Autodesk Inventor part; units mm, degrees
ref_plane "YZ Plane" through (0, 0, 0) normal (1, 0, 0) x (0, 1, 0)
ref_plane "XZ Plane" through (0, 0, 0) normal (0, 1, 0) x (-1, 0, 0)
ref_plane "XY Plane" through (0, 0, 0) normal (0, 0, 1) x (1, 0, 0)
sketch "Sketch1" plane through (0, 0, 0) normal (0, 1, 0) x (-1, 0, 0)
  line L0 (35, 45.5) -> (35, 15.5)
  line L1 (9, 15.5) -> (35, 15.5) construction
  line L2 (0, 15.5) -> (9, 15.5) construction
  line L3 (35, 15.5) -> (48, 15.5)
  line L4 (0, -45.5) -> (0, 45.5)
  line L5 (0, -45.5) -> (48, -45.5)
  line L6 (0, 45.5) -> (35, 45.5)
  line L7 (48, -45.5) -> (48, 15.5)
  line L8 (30.7, 40.55) -> (35, 40.55) construction
  line L9 (30.7, 40.55) -> (30.7, 22.45) construction
  circle A0 centre (30.7, 22.45) radius 1.25
  circle A1 centre (30.7, 40.55) radius 1.25
  line L10 (30.7, 22.45) -> (30.7, 15.5) construction
  line L11 (44, 15.5) -> (44, 9.5) construction
  line L12 (44, 9.5) -> (48, 9.5) construction
  circle A2 centre (44, 9.5) radius 1.25
  circle A3 centre (44, -28.5) radius 1.25
  circle A4 centre (18, -28.5) radius 1.25
  circle A5 centre (18, -38.5) radius 1.25
  arc A6 (0, -18.75) -> (0, -16.25) centre (0, -17.5) ccw
  arc A7 (0, 40.55) -> (0, 43.05) centre (0, 41.8) ccw
  arc A8 (0, 18.95) -> (0, 21.45) centre (0, 20.2) ccw
  line L13 (0, 41.8) -> (30.7, 41.8) construction
  circle A9 centre (40, -36.5) radius 6
  point P0 (0, 0)
  point P1 (-50, 0)
  point P2 (0, 0)
  dimension "d17" = 2.5
  dimension "d6" = 30
  dimension "d9" = 26
  dimension "d10" = 9
  dimension "d11" = 48
  dimension "d12" = 91
  dimension "d14" = 4.3
  dimension "d15" = 18.1
  dimension "d16" = 2.5
  dimension "d20" = 6.95
  dimension "d25" = 6
  dimension "d26" = 4
  dimension "d27" = 2.5
  dimension "d30" = 2.5
  dimension "d32" = 2.5
  dimension "d33" = 18
  dimension "d34" = 2.5
  dimension "d35" = 10
  dimension "d36" = 2.5
  dimension "d37" = 2.5
  dimension "d38" = 1.25
  dimension "d42" = 12
  dimension "d43" = 8
  dimension "d45" = 27
  dimension "d46" = 46
  dimension "d47" = 38
  dimension "d48" = 2.25
extrude "Extrusion1" add sketch "Sketch1" along normal blind 2 contours L0 L3 L7 L5 L4 A6 A8 A7 L6 | A7 L4 | A8 L4 | L4 A6 | A0 | A1 | A2 | A3 | A4 | A5 | A9
extrude "Extrusion2" cut sketch "Sketch1" along normal through all contours A7 L4 | A8 L4 | L4 A6 | A0 | A1 | A2 | A3 | A4 | A5 | A9
mirror "Mirror1" about plane through (0, 0, 0) normal (1, 0, 0) of "Extrusion1", "Extrusion2"
sketch "Sketch3" plane through (0, 0, 0) normal (1, 0, 0) x (0, 1, 0)
  line L0 (0, 15.5) -> (0, -45.5)
  line L1 (0, -45.5) -> (2, -45.5)
  line L2 (0, -45.5) -> (2, -45.5)
  line L3 (2, -45.5) -> (0, -43.5)
  line L4 (0, -43.5) -> (0, -45.5)
  line L5 (2, -45.5) -> (2, 15.5)
  point P0 (0, 0)
  dimension "d24" = 45
extrude "Extrusion3" cut sketch "Sketch3" along normal through all both and the other way through all
chamfer "Chamfer1" distance 2 angle 45 2 edges at (-41.5, 0, 15.5) (41.5, 0, 15.5)
properties part number "Podstawa"
Source: CAD feature listing. Evaluate the final solid. Frame: model axes, mm. Round coordinates to 2 decimals unless told otherwise and drop trailing zeros. Loops run counter-clockwise (first coordinate to the right, second up) from the corner with the lowest first, then second, coordinate; pieces in that order, holes last. Notation, with made-up numbers: M 42,-2 L 61,-2 A21 cw 61,27 Z; hole C -38.5,74 d4. An arc over 180 degrees is marked long. Use a Markdown table: item, result. Add a question column.
1. Cut plane C-C, the plane z = -38.5. Output: boundary loops of the cut face in (x, y).
2. Contact query for flat-ended pins moving along their axis: pin 1 (4 mm diameter, centred on x = -44, z = -28.5, fed in from +Y); pin 2 (0.6 mm diameter, centred on y = 0.5, z = 30, fed in from -X); pin 3 (2 mm diameter, centred on x = 0, z = 41.8, fed in from +Y). Output: stop coordinate, or through.
3. Cut plane A-A, the plane z = 9.5. Output: boundary loops of the cut face in (x, y).
4. Pull-direction query (X, two-part tool) for faces 1 (the flat face through (-48, 1, -15)), 2 (the flat face through (35, 1, 29)), 3 (the cylindrical face through (19.155, 0.986, -28.979)), 4 (the flat face through (41.4, 1, 14.5)); classes: +X half, -X half, draft (parallel to the pull), parting line (faces both ways), or undercut.
5. Ray query, line 1 along Z through (x, y) = (0, 0.75); line 2 along X through (y, z) = (0.9, -27.5); line 3 along Z through (x, y) = (-18, 1.35). Return the intervals inside material, ascending. Write a range as [from, to].
6. Cut plane B-B, the plane x = 30.7. Output: boundary loops of the cut face in (y, z), and give its area (3 significant figures).
7. Cut plane D-D, the plane y = 1. State how many separate pieces and enclosed holes the cut face has, and give its area (3 significant figures).
Solution:
| question | item | result |
|---|---|---|
| 1 | outline | M -48,0 L -45.66,0 L -45.66,2 L -48,2 Z; M -34.34,0 L -19.25,0 L -19.25,2 L -34.34,2 Z; M -16.75,0 L 16.75,0 L 16.75,2 L -16.75,2 Z; M 19.25,0 L 34.34,0 L 34.34,2 L 19.25,2 Z; M 45.66,0 L 48,0 L 48,2 L 45.66,2 Z |
| 2 | pin 1 | stops at y = 2 |
| 2 | pin 2 | stops at x = -35 |
| 2 | pin 3 | passes through |
| 3 | outline | M -48,0 L -45.25,0 L -45.25,2 L -48,2 Z; M -42.75,0 L 42.75,0 L 42.75,2 L -42.75,2 Z; M 45.25,0 L 48,0 L 48,2 L 45.25,2 Z |
| 4 | face 1 | -X half |
| 4 | face 2 | +X half |
| 4 | face 3 | undercut |
| 4 | face 4 | draft |
| 5 | line 1 | z = [-44.25, -18.75], [-16.25, 18.95], [21.45, 40.55], [43.05, 45.5] |
| 5 | line 2 | x = [-48, -44.75], [-43.25, -18.75], [-17.25, 17.25], [18.75, 43.25], [44.75, 48] |
| 5 | line 3 | z = [-44.85, -39.75], [-37.25, -29.75], [-27.25, 45.5] |
| 6 | outline | M 0,-43.5 L 2,-45.5 L 2,21.2 L 0,21.2 Z; M 0,23.7 L 2,23.7 L 2,39.3 L 0,39.3 Z; M 0,41.8 L 2,41.8 L 2,45.5 L 0,45.5 Z |
| 6 | area | 170 mm2 |
| 7 | separate pieces | 1 |
| 7 | enclosed holes | 17 |
| 7 | area | 7,530 mm2 |
